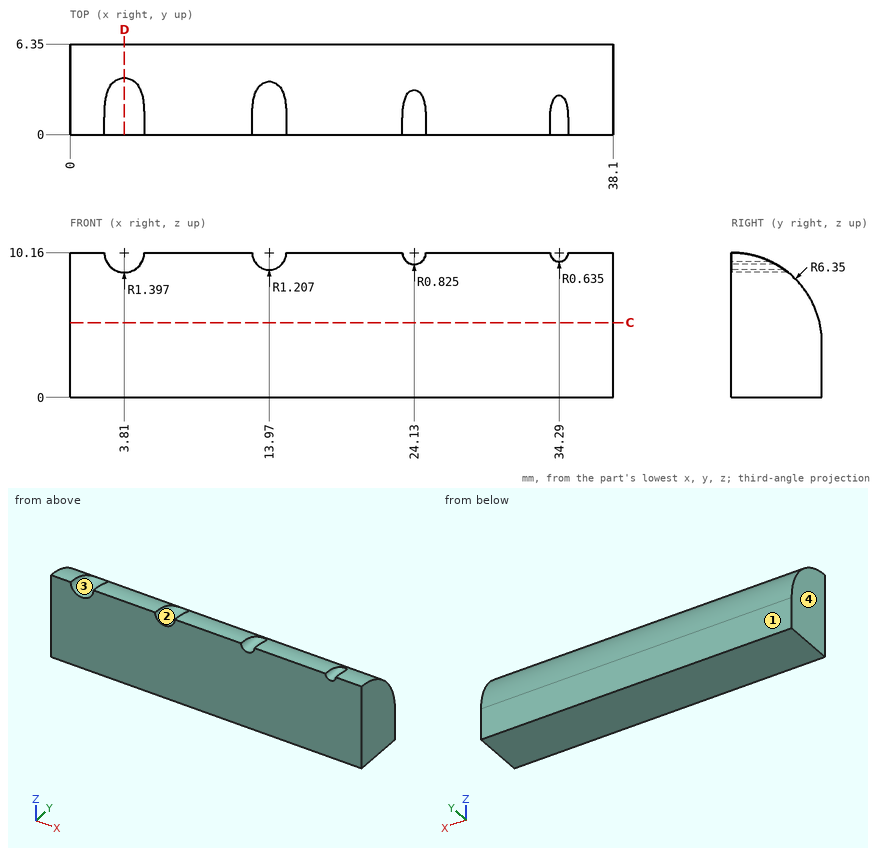
Answer from the drawing. Dimensions are ordinates in mm from the lowest x, y and z of the part. Give positions to 0.01 mm unless a question says otherwise; leave off trailing zeros. Order: outer loops, then holes, each group sorted by start corner. A loop starts at its lowest first (then second) coordinate and runs counter-clockwise, first axis right, second up. Notation, with made-up numbers: (14.5, 10) - (61.5, 10) arc R24 cw to (61.5, 37) - close; hole circle Ø7 at (-32.75, 4). An arc over 180 degrees is marked (long way). One line per item, written item: value. Start each with the question number.
1) The mould has two halves that part along X. Classify the marked faces 1, 2, 3 and 4: released by +X, released by -X, zero draft, split by the parting line, or undercut.
2) Find the intervals of material crossed by L1, parallel to Y at x = 32, z = 4; L2, parallel to Z at x = 23.5, y = 2.25 (1 decimal); L3, parallel to Z at x = 12, y = 3.5, in increasing order.
3) A cutting plane is placed at C-C on z = 5.25. Give the vertices of the cut face in (x, y) (1 decimal).
4) A cutting plane is placed at D-D on x = 3.81. Give the vertices of the cut face in (y, z).
5) Given pin 1 Ø3 at (x, z) = (4, 7) entering from +Y; pin 2 Ø1 at (x, z) = (10.5, 7.5) entering from +Y, each flat-ended and moving along its own axis, determine where each tip first touches the part or whether it passes through.
Answer sheet:
1. face 1: zero draft
1. face 2: undercut
1. face 3: undercut
1. face 4: released by -X
2. L1: y = 0 to 6.35
2. L2: z = 0 to 9.6
2. L3: z = 0 to 9.11
3. outline: (0, 0) - (38.1, 0) - (38.1, 6.2) - (0, 6.2) - close
4. outline: (0, 0) - (6.35, 0) - (6.35, 3.81) arc R6.35 ccw to (3.97, 8.76) - (0, 8.76) - close
5. pin 1: stops at y = 6.12
5. pin 2: stops at y = 5.49
